Part print with two shaded views. Sizes in mm from the minimum x, y, z corner. Round coordinates to 2 decimals unless told otherwise and drop trailing zeros. Loops run counter-clockwise (first coordinate to the right, second up) from the corner with the lowest first, then second, coordinate; pieces in that order, holes last.
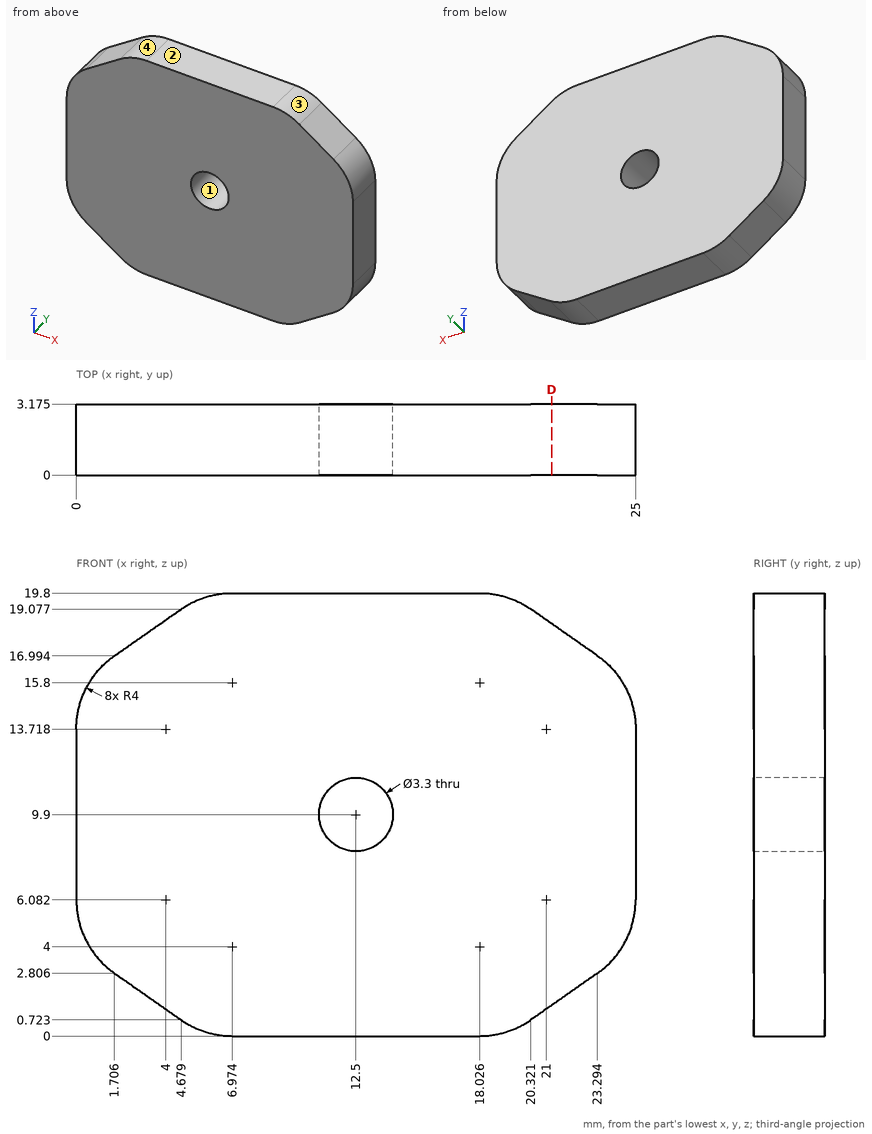
Item 1: Cut at D-D (x = 21.25). List the corners of the cut face in (y, z) (1 decimal).
Verdict:
outline: (0, 1.4) - (3.2, 1.4) - (3.2, 18.4) - (0, 18.4) - close
Item 2: Mould opens along X. For the marked faces 1, 2, 3 and 4 say: released by +X, released by -X, zero draft, split by the parting line, or undercut.
Verdict:
face 1: undercut
face 2: zero draft
face 3: released by +X
face 4: released by -X
Item 3: Flat gauge pin, fed straight in: P1, Ø6, axis at x = 13.5, z = 11, coming from the -Y side. Where does the tip first touch, or does it go through?
Verdict:
P1: stops at y = 0
Item 4: Wall check: L1, parallel to X at y = 1.5, z = 9.9; L2, parallel to X at y = 0.85, z = 10.5; L3, parallel to Z at x = 21.75, y = 1.5 (1 decimal). Give the ranges that are in metal, low to high.
Verdict:
L1: x = 0 to 10.85, 14.15 to 25
L2: x = 0 to 10.96, 14.04 to 25
L3: z = 1.7 to 18.1
